from build123d import *

# Parameters (mm, degrees)
F0_W     = 60
F0_H     = 150
F1_DEPTH = 3
F2_R     = 6
F2_R_2   = 4
F3_DEPTH = 290
F5_D     = 5


with BuildPart() as f1:
    # F0 (on Front) → F1 (new body)
    with BuildSketch(Plane.XZ):
        Rectangle(F0_W, F0_H)
    extrude(amount=F1_DEPTH)

    # F2 (on face) → F3 (join)
    with BuildSketch(Plane.XZ.offset(3)):
        Circle(F2_R)
        Circle(F2_R_2, mode=Mode.SUBTRACT)
    extrude(amount=F3_DEPTH)

    # F5 (through all)
    with Locations(Plane.XZ.offset(3)):
        with Locations((-20, 65), (0, 65), (20, 65), (20, -65), (0, -65), (-20, -65)):
            Hole(F5_D / 2)


solid = f1.part
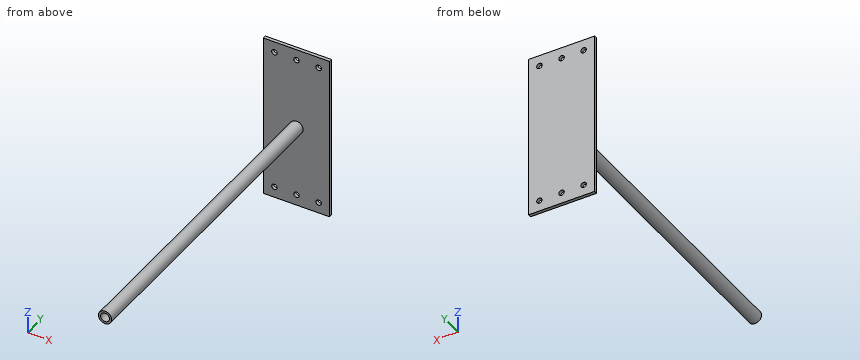
Work out the finished part from the listing and answer in its coordinate system (mm). Give positions to 0.01 mm unless a question says otherwise; leave off trailing zeros. Write each loop counter-clockwise with the first axis right and the second up, starting at its lowest first coordinate (ties: lowest second). Pieces come first, ordered by that corner, then holes. Notation, with made-up numbers: M 23.5,-37 L 79.5,-37 A5 cw 79.5,-31 Z; hole C 1,67.5 d1. An arc over 180 degrees is marked long. Answer as CSV lines item,"result".
Q1. Given P1, Ø6.5, axis at x = 20, z = -65, coming from the -Y side; P2, Ø12, axis at y = -233, z = 7, coming from the -X side, each flat-ended and moving along its own axis, determine where each tip first touches the part or whether it passes through.
A:
P1,"stops at y = -3"
P2,"stops at x = -5.92"
Q2. Find the intervals of material crossed by probe 1 along Z at (x, y) = (-20, -1); probe 2 along Z at (x, y) = (0, -183); probe 3 along Y at (x, z) = (-12.5, 51), in increasing order. Write a range as [from, to].
A:
probe 1,"z = [-75, -67.5], [-62.5, 62.5], [67.5, 75]"
probe 2,"z = [-6, -4], [4, 6]"
probe 3,"y = [-3, 0]"
Q3. A cutting plane is placed at B-B on z = -59.5. Write down the section's boundary in (x, y), plus the area to 3 significant figures.
A:
outline,"M -30,-3 L 30,-3 L 30,0 L -30,0 Z"
area,"180 mm²"
Q4. A cutting plane is placed at A-A on y = -195.5. Write down the section's boundary in (x, z), plus the area to 3 significant figures.
A:
outline,"C 0,0 d12; hole C 0,0 d8"
area,"62.8 mm²"
